Solid Edge part; units mm, degrees
sketch "Sketch1" plane through (0, 0, 0) normal (0, 0, 1) x (1, 0, 0)
  line L0 (-20.7402, -11.3602) -> (4.2598, -11.3602)
  line L1 (4.2598, -11.3602) -> (4.2598, -8.3602)
  line L2 (4.2598, -8.3602) -> (-5.2402, -5.3602)
  line L3 (-5.2402, -5.3602) -> (-11.2402, -5.3602)
  line L4 (-20.7402, -8.3602) -> (-11.2402, -5.3602)
  line L5 (-20.7402, -8.3602) -> (-20.7402, -11.3602)
extrude "Protrusion1" add sketch "Sketch1" along normal blind 25
sketch "Sketch2" plane through (4.2598, -9.8602, 12.5) normal (1, 0, 0) x (0, 0, -1)
  line L0 (-12.5, 1.5) -> (-3, 4.5181)
  line L1 (-3, 4.5181) -> (2.994, 4.5)
  line L2 (2.994, 4.5) -> (12.5, 1.5)
extrude "Cutout1" cut sketch "Sketch2" against normal through all material side at (4.2598, -6.8035, 20.2651)
sketch "Sketch3" plane through (-5.2402, 0, 0) normal (1, 0, 0) x (0, 1, 0)
  circle A0 centre (4.1398, 12.5698) radius 11.592
  circle A1 centre (4.1398, 12.5698) radius 9.4412
extrude "ExtrudedProtrusion_2" add sketch "Sketch3" against normal blind 6.35
CAD build for the part. Positions are in the model's coordinates, mm. Coordinates: 2 decimals unless noted, no trailing zeros. Write each loop counter-clockwise with the first axis right and the second up, starting at its lowest first coordinate (ties: lowest second). Pieces come first, ordered by that corner, then holes. Notation, with made-up numbers: (-36, -11.75) -> (-31, -11.75) arc R23 cw to (-31, 26.25) -> close; hole circle Ø9 at (22.5, 42.25). An arc over 180 degrees is marked (long way). Return JSON: item names as keys, results as strings. Group by question number.
Q1. Flat gauge pins, fed straight in: pin 1 (6 mm diameter, centred on y = 10, z = 10, fed in from -X); pin 2 (1.5 mm diameter, centred on y = 1, z = 4, fed in from -X); pin 3 (8 mm diameter, centred on y = 11, z = 4.5, fed in from +X); pin 4 (1.5 mm diameter, centred on x = -16, z = 3, fed in from +Y). Where does each tip first touch, or does it go through?
Q2. Cut at C-C, the plane z = 11.5. Give the cut face in (x, y), then the cut area to 3 significant figures.
Q3. Cut at B-B, the plane z = 19.25. Give the cut face in (x, y), then the cut area to 3 significant figures.
Q4. Drill centre lines: line 1 (Y direction, x = -5.5, z = 12.5); line 2 (Y direction, x = -10.75, z = 7.5); line 3 (X direction, y = -4, z = 5.5). Where is each one in solid material? Low to high.
Q5. Pull direction Y, two halves, no side cores. Call faces 1 (the face through (-8.065, -7.173, 3.763)), 2 (the face through (-8, -10, 25)), 3 (the face through (-17.25, -7.26, 12.32)): released by +Y, released by -Y, zero draft, split by the parting line, or undercut.
Q6. Cut at A-A, the plane y = 2. Give the cut face in (x, z).
Q7. Cut at D-D, the plane x = -8. Give the cut face in (y, z).
Returned:
{
 "1": {"pin 1": "passes through", "pin 2": "stops at x = -11.59", "pin 3": "stops at x = -5.24", "pin 4": "stops at y = -7.18"},
 "2": {"outline": "(-20.74, -11.36) -> (4.26, -11.36) -> (4.26, -8.36) -> (-5.24, -5.36) -> (-5.24, -5.24) -> (-11.59, -5.24) -> (-11.59, -5.47) -> (-20.74, -8.36) -> close; (-11.59, 13.52) -> (-5.24, 13.52) -> (-5.24, 15.68) -> (-11.59, 15.68) -> close", "area": "136 mm2"},
 "3": {"outline": "(-20.74, -11.36) -> (4.26, -11.36) -> (4.26, -8.36) -> (-1.52, -6.53) -> (-14.96, -6.53) -> (-20.74, -8.36) -> close; (-11.59, -5.33) -> (-5.24, -5.33) -> (-5.24, -2.53) -> (-11.59, -2.53) -> close; (-11.59, 10.81) -> (-5.24, 10.81) -> (-5.24, 13.61) -> (-11.59, 13.61) -> close", "area": "146 mm2"},
 "4": {"line 1": "y = -11.36 to -5.3, 13.58 to 15.73", "line 2": "y = -11.36 to -3.82, 12.1 to 14.56", "line 3": "x = -11.59 to -5.24"},
 "5": {"face 1": "undercut", "face 2": "zero draft", "face 3": "released by +Y"},
 "6": {"outline": "(-11.59, 1.18) -> (-5.24, 1.18) -> (-5.24, 3.37) -> (-11.59, 3.37) -> close; (-11.59, 21.77) -> (-5.24, 21.77) -> (-5.24, 23.96) -> (-11.59, 23.96) -> close"},
 "7": {"outline": "(-11.36, 0) -> (-8.36, 0) -> (-6.11, 7.15) arc R11.59 ccw (long way) to (-6.12, 17.96) -> (-8.36, 25) -> (-11.36, 25) -> close; hole circle Ø18.88 at (4.14, 12.57)"}
}
